Source: three-view drawing plus pictorial views. Frame: mm from the lowest corner of the part. Give positions to 0.01 mm unless a question says otherwise; leave off trailing zeros. Loops run counter-clockwise (first coordinate to the right, second up) from the corner with the lowest first, then second, coordinate; pieces in that order, holes last. Notation, with made-up numbers: (65, 29.5) - (124, 29.5) arc R13 ccw to (124, 47.5) - close; hole circle Ø1 at (13.25, 3.5). An arc over 180 degrees is marked (long way). Write each question's results on one line, items separated by ' | '. Start each with the question number.
(1) Cut plane D-D on z = 7.5. Return the cut outline in (x, y), then the cut area to 3 significant figures.
(2) Cut plane A-A on x = 11. Return the cut outline in (y, z).
(3) Cut plane B-B on z = 11. Return the cut outline in (x, y), then the cut area to 3 significant figures.
(4) Pull-direction query (X, two-part tool) for the marked faces 1, 2 and 3; classes: pulls with the +X half, pulls with the -X half, needs draft (parallel to the pull), parting line crosses it, or undercut.
(5) Contact query for flat-ended pins moving along their axis: pin 1 (1.5 mm diameter, centred on y = 41, z = 14, fed in from -X); pin 2 (6 mm diameter, centred on x = 7.5, y = 54.5, fed in from -Z); pin 3 (1 mm diameter, centred on y = 15.5, z = 5, fed in from +X). Output: stop coordinate, or through.
(6) Cut plane C-C on y = 27. Return the cut outline in (x, z), then the cut area to 3 significant figures.
(7) Material intervals for line 1 along X through (y, z) = (53, 11); line 2 along X through (y, z) = (35.4, 11); line 3 along Y through (x, z) = (5.5, 9), sorted ascending. Write a range as [from, to].
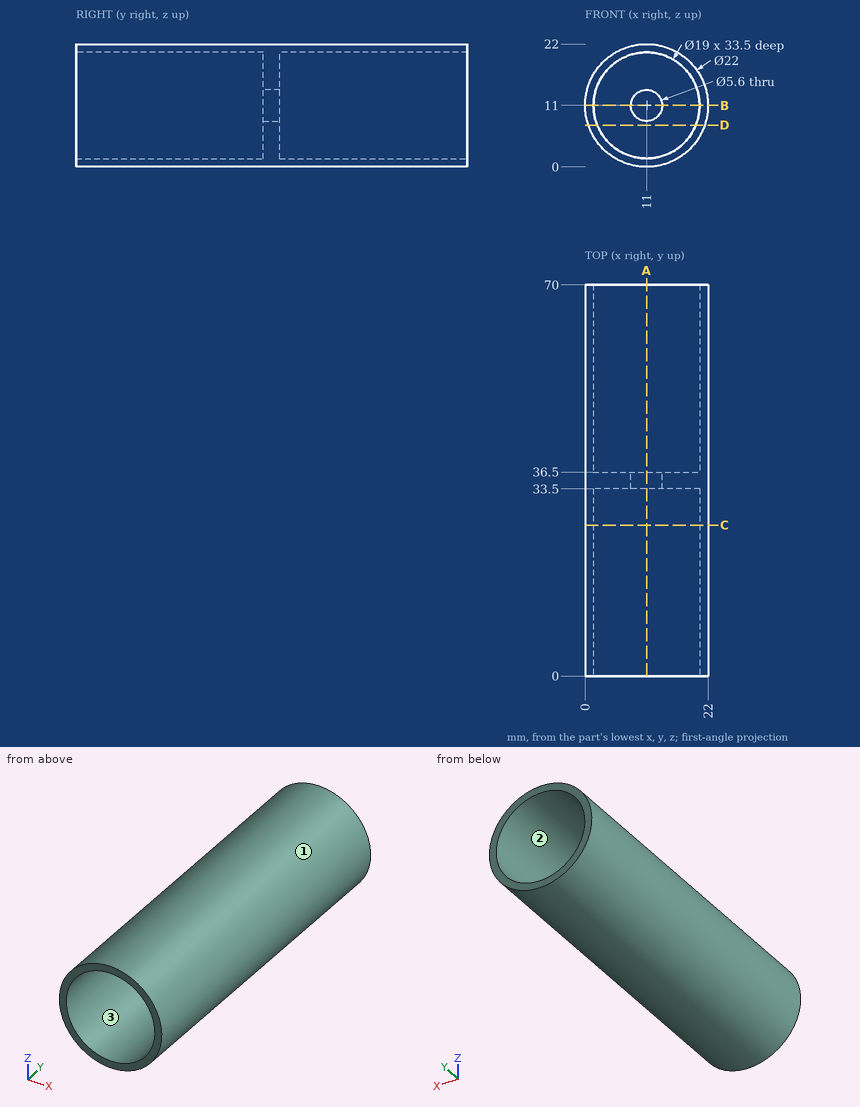
Ans:
1) outline: (0.57, 0) - (2.17, 0) - (2.17, 33.5) - (19.83, 33.5) - (19.83, 0) - (21.43, 0) - (21.43, 70) - (19.83, 70) - (19.83, 36.5) - (2.17, 36.5) - (2.17, 70) - (0.57, 70) - close | area: 277 mm^2
2) outline: (0, 0) - (70, 0) - (70, 1.5) - (36.5, 1.5) - (36.5, 8.2) - (33.5, 8.2) - (33.5, 1.5) - (0, 1.5) - close; (0, 20.5) - (33.5, 20.5) - (33.5, 13.8) - (36.5, 13.8) - (36.5, 20.5) - (70, 20.5) - (70, 22) - (0, 22) - close
3) outline: (0, 0) - (1.5, 0) - (1.5, 33.5) - (8.2, 33.5) - (8.2, 36.5) - (1.5, 36.5) - (1.5, 70) - (0, 70) - close; (13.8, 33.5) - (20.5, 33.5) - (20.5, 0) - (22, 0) - (22, 70) - (20.5, 70) - (20.5, 36.5) - (13.8, 36.5) - close | area: 250 mm^2
4) face 1: parting line crosses it | face 2: undercut | face 3: undercut
5) pin 1: x = 0.23 | pin 2: z = 0.01 | pin 3: x = 20.53
6) outline: circle Ø22 at (11, 11); hole circle Ø19 at (11, 11) | area: 96.6 mm^2
7) line 1: [0, 1.5], [20.5, 22] | line 2: [0, 8.2], [13.8, 22] | line 3: [33.5, 36.5]
